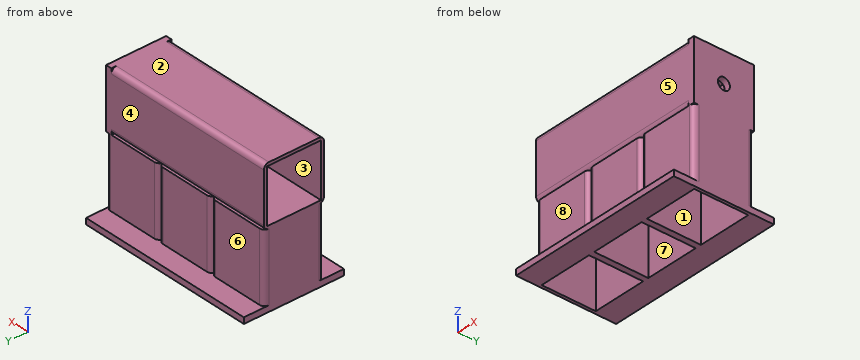
from build123d import *

# Parameters (mm, degrees)
F0_W     = 54
F0_H     = 54
F1_DEPTH = 69
F2_W     = 54
F2_H     = 54
F3_DEPTH = 6
F4_W     = 54
F4_H     = 54
F5_DEPTH = 180
F6_W     = 60
F6_H     = 60
F6_R     = 6
F7_DEPTH = 6


with BuildPart() as f1:
    # F0 (on Top) → F1 (new body)
    with BuildSketch(Plane.XY):
        with BuildLine():
            ThreePointArc((-10.85040465, -8.5986092687), (-12.314870744, -5.0630753627), (-15.85040465, -3.5986092687))
            Line((-15.85040465, -3.5986092687), (-65.85040465, -3.5986092687))
            ThreePointArc((-65.85040465, -3.5986092687), (-69.3859385559, -5.0630753627), (-70.85040465, -8.5986092687))
            Line((-70.85040465, -8.5986092687), (-70.85040465, -58.5986092687))
            ThreePointArc((-70.85040465, -58.5986092687), (-69.3859385559, -62.1341431746), (-65.85040465, -63.5986092687))
            Line((-65.85040465, -63.5986092687), (-15.85040465, -63.5986092687))
            ThreePointArc((-15.85040465, -63.5986092687), (-12.314870744, -62.1341431746), (-10.85040465, -58.5986092687))
            Line((-10.85040465, -58.5986092687), (-10.85040465, -8.5986092687))
        make_face()
        with Locations((-40.85040465, -33.5986092687)):
            Rectangle(F0_W, F0_H, mode=Mode.SUBTRACT)
        with BuildLine():
            ThreePointArc((-5.85040465, -3.5986092687), (-9.3859385559, -5.0630753627), (-10.85040465, -8.5986092687))
            Line((-10.85040465, -8.5986092687), (-10.85040465, -58.5986092687))
            ThreePointArc((-10.85040465, -58.5986092687), (-9.3859385559, -62.1341431746), (-5.85040465, -63.5986092687))
            Line((-5.85040465, -63.5986092687), (44.14959535, -63.5986092687))
            ThreePointArc((44.14959535, -63.5986092687), (47.685129256, -62.1341431746), (49.14959535, -58.5986092687))
            Line((49.14959535, -58.5986092687), (49.14959535, -8.5986092687))
            ThreePointArc((49.14959535, -8.5986092687), (47.685129256, -5.0630753627), (44.14959535, -3.5986092687))
            Line((44.14959535, -3.5986092687), (-5.85040465, -3.5986092687))
        make_face()
        with Locations((19.14959535, -33.5986092687)):
            Rectangle(F0_W, F0_H, mode=Mode.SUBTRACT)
        with BuildLine():
            ThreePointArc((54.14959535, -3.5986092687), (50.6140614441, -5.0630753627), (49.14959535, -8.5986092687))
            Line((49.14959535, -8.5986092687), (49.14959535, -58.5986092687))
            ThreePointArc((49.14959535, -58.5986092687), (50.6140614441, -62.1341431746), (54.14959535, -63.5986092687))
            Line((54.14959535, -63.5986092687), (104.14959535, -63.5986092687))
            ThreePointArc((104.14959535, -63.5986092687), (107.685129256, -62.1341431746), (109.14959535, -58.5986092687))
            Line((109.14959535, -58.5986092687), (109.14959535, -8.5986092687))
            ThreePointArc((109.14959535, -8.5986092687), (107.685129256, -5.0630753627), (104.14959535, -3.5986092687))
            Line((104.14959535, -3.5986092687), (54.14959535, -3.5986092687))
        make_face()
        with Locations((79.14959535, -33.5986092687)):
            Rectangle(F0_W, F0_H, mode=Mode.SUBTRACT)
    extrude(amount=F1_DEPTH)

    # F2 (on face) → F3 (join)
    with BuildSketch(Plane(origin=(0, 0, 0), x_dir=(1, 0, 0), z_dir=(0, 0, -1))):
        with BuildLine():
            Line((-70.85040465, -16.4013907313), (109.14959535, -16.4013907313))
            Line((109.14959535, -16.4013907313), (109.14959535, 8.5986092687))
            ThreePointArc((109.14959535, 8.5986092687), (107.685129256, 5.0630753627), (104.14959535, 3.5986092687))
            Line((104.14959535, 3.5986092687), (54.14959535, 3.5986092687))
            ThreePointArc((54.14959535, 3.5986092687), (50.6140614441, 5.0630753627), (49.14959535, 8.5986092687))
            ThreePointArc((49.14959535, 8.5986092687), (47.685129256, 5.0630753627), (44.14959535, 3.5986092687))
            Line((44.14959535, 3.5986092687), (-5.85040465, 3.5986092687))
            ThreePointArc((-5.85040465, 3.5986092687), (-9.3859385559, 5.0630753627), (-10.85040465, 8.5986092687))
            ThreePointArc((-10.85040465, 8.5986092687), (-12.314870744, 5.0630753627), (-15.85040465, 3.5986092687))
            Line((-15.85040465, 3.5986092687), (-65.85040465, 3.5986092687))
            ThreePointArc((-65.85040465, 3.5986092687), (-69.3859385559, 5.0630753627), (-70.85040465, 8.5986092687))
            Line((-70.85040465, 8.5986092687), (-70.85040465, -16.4013907313))
        make_face()
        with BuildLine():
            ThreePointArc((104.14959535, 63.5986092687), (107.685129256, 62.1341431746), (109.14959535, 58.5986092687))
            Line((109.14959535, 58.5986092687), (109.14959535, 83.5986092687))
            Line((109.14959535, 83.5986092687), (-70.85040465, 83.5986092687))
            Line((-70.85040465, 83.5986092687), (-70.85040465, 58.5986092687))
            ThreePointArc((-70.85040465, 58.5986092687), (-69.3859385559, 62.1341431746), (-65.85040465, 63.5986092687))
            Line((-65.85040465, 63.5986092687), (-15.85040465, 63.5986092687))
            ThreePointArc((-15.85040465, 63.5986092687), (-12.314870744, 62.1341431746), (-10.85040465, 58.5986092687))
            ThreePointArc((-10.85040465, 58.5986092687), (-9.3859385559, 62.1341431746), (-5.85040465, 63.5986092687))
            Line((-5.85040465, 63.5986092687), (44.14959535, 63.5986092687))
            ThreePointArc((44.14959535, 63.5986092687), (47.685129256, 62.1341431746), (49.14959535, 58.5986092687))
            ThreePointArc((49.14959535, 58.5986092687), (50.6140614441, 62.1341431746), (54.14959535, 63.5986092687))
            Line((54.14959535, 63.5986092687), (104.14959535, 63.5986092687))
        make_face()
        with BuildLine():
            ThreePointArc((104.14959535, 3.5986092687), (107.685129256, 5.0630753627), (109.14959535, 8.5986092687))
            Line((109.14959535, 8.5986092687), (109.14959535, 58.5986092687))
            ThreePointArc((109.14959535, 58.5986092687), (107.685129256, 62.1341431746), (104.14959535, 63.5986092687))
            Line((104.14959535, 63.5986092687), (54.14959535, 63.5986092687))
            ThreePointArc((54.14959535, 63.5986092687), (50.6140614441, 62.1341431746), (49.14959535, 58.5986092687))
            ThreePointArc((49.14959535, 58.5986092687), (47.685129256, 62.1341431746), (44.14959535, 63.5986092687))
            Line((44.14959535, 63.5986092687), (-5.85040465, 63.5986092687))
            ThreePointArc((-5.85040465, 63.5986092687), (-9.3859385559, 62.1341431746), (-10.85040465, 58.5986092687))
            ThreePointArc((-10.85040465, 58.5986092687), (-12.314870744, 62.1341431746), (-15.85040465, 63.5986092687))
            Line((-15.85040465, 63.5986092687), (-65.85040465, 63.5986092687))
            ThreePointArc((-65.85040465, 63.5986092687), (-69.3859385559, 62.1341431746), (-70.85040465, 58.5986092687))
            Line((-70.85040465, 58.5986092687), (-70.85040465, 8.5986092687))
            ThreePointArc((-70.85040465, 8.5986092687), (-69.3859385559, 5.0630753627), (-65.85040465, 3.5986092687))
            Line((-65.85040465, 3.5986092687), (-15.85040465, 3.5986092687))
            ThreePointArc((-15.85040465, 3.5986092687), (-12.314870744, 5.0630753627), (-10.85040465, 8.5986092687))
            ThreePointArc((-10.85040465, 8.5986092687), (-9.3859385559, 5.0630753627), (-5.85040465, 3.5986092687))
            Line((-5.85040465, 3.5986092687), (44.14959535, 3.5986092687))
            ThreePointArc((44.14959535, 3.5986092687), (47.685129256, 5.0630753627), (49.14959535, 8.5986092687))
            ThreePointArc((49.14959535, 8.5986092687), (50.6140614441, 5.0630753627), (54.14959535, 3.5986092687))
            Line((54.14959535, 3.5986092687), (104.14959535, 3.5986092687))
        make_face()
        with Locations((-40.85040465, 33.5986092687)):
            Rectangle(F2_W, F2_H, mode=Mode.SUBTRACT)
        with Locations((19.14959535, 33.5986092687)):
            Rectangle(F2_W, F2_H, mode=Mode.SUBTRACT)
        with Locations((79.14959535, 33.5986092687)):
            Rectangle(F2_W, F2_H, mode=Mode.SUBTRACT)
    extrude(amount=F3_DEPTH)

    # F4 (on face) → F5 (join, through all)
    with BuildSketch(Plane.YZ.offset(109.14959535)):
        with BuildLine():
            ThreePointArc((-3.5986092687, 124), (-5.0630753627, 127.5355339059), (-8.5986092687, 129))
            Line((-8.5986092687, 129), (-58.5986092687, 129))
            ThreePointArc((-58.5986092687, 129), (-62.1341431746, 127.5355339059), (-63.5986092687, 124))
            Line((-63.5986092687, 124), (-63.5986092687, 74))
            ThreePointArc((-63.5986092687, 74), (-62.1341431746, 70.4644660941), (-58.5986092687, 69))
            Line((-58.5986092687, 69), (-8.5986092687, 69))
            ThreePointArc((-8.5986092687, 69), (-5.0630753627, 70.4644660941), (-3.5986092687, 74))
            Line((-3.5986092687, 74), (-3.5986092687, 124))
        make_face()
        with Locations((-33.5986092687, 99)):
            Rectangle(F4_W, F4_H, mode=Mode.SUBTRACT)
    extrude(amount=-F5_DEPTH)

    # F6 (on face) → F7 (join)
    with BuildSketch(Plane.YZ.offset(109.14959535)):
        with Locations((-33.5986092687, 99)):
            Rectangle(F6_W, F6_H)
        with Locations((-33.5986092687, 99)):
            Circle(F6_R, mode=Mode.SUBTRACT)
    extrude(amount=-F7_DEPTH)


solid = f1.part
Verification items for the finished model (mm, model axes). Face numbers are marked on the shaded views. A direction names the side the tool comes from. Give positions to 0.01 mm unless a question says otherwise; leave off trailing zeros. Write each loop counter-clockwise with the first axis right and the second up, starting at its lowest first coordinate (ties: lowest second). Pieces come first, ordered by that corner, then holes. Notation, with made-up numbers: (-27.75, 22.25) - (-23.75, 22.25) arc R18 ccw to (-23.75, 57.25) - close; hole circle Ø6 at (-2, 10). An arc over 180 degrees is marked (long way). Answer as CSV lines item,"result". Start each with the question number.
1. Sectioned sample at B-B (z = 99). Record the boundary of the cut face in (x, y), then the cut area to 3 significant figures.
2. Sectioned sample at A-A (x = -45). Record the boundary of the cut face in (y, z).
3. Draft check along Y on the marked faces 6, 7 and 8. Enter one of: pulls with the +Y half, pulls with the -Y half, needs draft (parallel to the pull), parting line crosses it, or undercut.
4. Depth check by flat-ended pin: pin 1 (25 mm diameter, centred on x = 8.5, z = 26.5, fed in from -Y); pin 2 (4 mm diameter, centred on x = 5, z = 58, fed in from +Y); pin 3 (1.5 mm diameter, centred on x = 14.5, y = -5.5, fed in from +Z). Enter the tip coordinate at first touch or a pass-through.
5. Sectioned sample at C-C (z = 66.5). Count the separate pieces of the cut face and the enclosed holes in it, then the cut area to 3 significant figures.
6. Set-up check for the marked faces 1, 2, 3, 4 and 5: record each of +Z, -Z, +X, -X, +Y, -Y from which the full face is reachable in a straight line by a thin tool's end or side.
7. Sectioned sample at D-D (y = -12.5). Record the boundary of the cut face in (x, z).
8. Thickness scan on line 1 (X direction, y = -40.5, z = 16.5); line 2 (Y direction, x = -52.5, z = 40.5); line 3 (Z direction, x = 14, y = -51.5). Record the ranges inside material, lowest first.
Derived:
1,outline,"(-70.85, -63.6) - (109.15, -63.6) - (109.15, -39.6) - (103.15, -39.6) - (103.15, -60.6) - (-70.85, -60.6) - close; (-70.85, -6.6) - (103.15, -6.6) - (103.15, -27.6) - (109.15, -27.6) - (109.15, -3.6) - (-70.85, -3.6) - close"
1,area,"1,330 mm²"
2,outline,"(-83.6, -6) - (-60.6, -6) - (-60.6, 69) - (-63.6, 69) - (-63.6, 0) - (-83.6, 0) - close; (-63.6, 74) arc R5 ccw to (-58.6, 69) - (-8.6, 69) arc R5 ccw to (-3.6, 74) - (-3.6, 124) arc R5 ccw to (-8.6, 129) - (-58.6, 129) arc R5 ccw to (-63.6, 124) - close; (-6.6, -6) - (16.4, -6) - (16.4, 0) - (-3.6, 0) - (-3.6, 69) - (-6.6, 69) - close; hole (-60.6, 72) - (-6.6, 72) - (-6.6, 126) - (-60.6, 126) - close"
3,face 6,"pulls with the +Y half"
3,face 7,"undercut"
3,face 8,"pulls with the -Y half"
4,pin 1,"y = -63.6"
4,pin 2,"y = -3.6"
4,pin 3,"z = 128.41"
5,separate pieces,"1"
5,enclosed holes,"3"
5,area,"1,990 mm²"
6,face 1,"-Z"
6,face 2,"+Z, +X, -X, +Y, -Y"
6,face 3,"-X"
6,face 4,"+Z, +X, -X, +Y"
6,face 5,"+Z, +X, -X, -Y"
7,outline,"(-70.85, -6) - (-67.85, -6) - (-67.85, 69) - (-13.85, 69) - (-13.85, -6) - (-7.85, -6) - (-7.85, 69) - (46.15, 69) - (46.15, -6) - (52.15, -6) - (52.15, 69) - (106.15, 69) - (106.15, -6) - (109.15, -6) - (109.15, 129) - (-70.85, 129) - (-70.85, 126) - (103.15, 126) - (103.15, 72) - (-70.85, 72) - close"
8,line 1,"-70.85 to -67.85, -13.85 to -7.85, 46.15 to 52.15, 106.15 to 109.15"
8,line 2,"-63.6 to -60.6, -6.6 to -3.6"
8,line 3,"69 to 72, 126 to 129"
